Autodesk Inventor part; units mm, degrees
ref_plane "YZ Plane" through (0, 0, 0) normal (1, 0, 0) x (0, 1, 0)
ref_plane "XZ Plane" through (0, 0, 0) normal (0, 1, 0) x (-1, 0, 0)
ref_plane "XY Plane" through (0, 0, 0) normal (0, 0, 1) x (1, 0, 0)
sketch "Sketch1" plane through (0, 0, 0) normal (0, 0, 1) x (1, 0, 0)
  line L0 (-25.4072, 25.3665) -> (76.1928, 25.3665)
  line L1 (76.1928, 25.3665) -> (76.1928, -76.2335)
  line L2 (76.1928, -76.2335) -> (-25.4072, -76.2335)
  line L3 (-25.4072, -76.2335) -> (-25.4072, 25.3665)
  point P0 (0, 0)
  dimension "d0" = 101.6
  dimension "d1" = 101.6
extrude "Extrusion1" add sketch "Sketch1" along normal blind 0.7366
sketch "Sketch2" plane through (0, 0, 0.7366) normal (0, 0, 1) x (1, 0, 0)
  line L0 (-25.4072, 25.3665) -> (76.1928, -76.2335)
  line L1 (76.1928, 25.3665) -> (-25.4072, -76.2335)
  circle A0 centre (25.3928, -25.4335) radius 27.432
  point P0 (0, 0)
  dimension "d4" = 54.864
extrude "Extrusion2" cut sketch "Sketch2" against normal blind 0.7366
sketch "Sketch3" plane through (0, 0, 0.7366) normal (0, 0, 1) x (1, 0, 0)
  line L0 (-25.4072, -76.2335) -> (-25.4072, 25.3665)
  line L1 (-25.4072, 25.3665) -> (-25.4072, -25.4335)
  line L2 (-25.4072, -25.4335) -> (-25.4072, 19.4102)
  line L3 (-25.4072, 25.3665) -> (76.1928, -76.2335)
  line L4 (76.1928, 25.3665) -> (-25.4072, -76.2335)
  circle A0 centre (-19.4509, 19.4102) radius 1.9812
  point P0 (0, 0)
  dimension "d7" = 44.8437
  dimension "d8" = 3.9624
extrude "Extrusion3" cut sketch "Sketch3" against normal blind 0.7366 contours A0 L3 | L3 A0
sketch "Sketch4" plane through (0, 0, 0.7366) normal (0, 0, 1) x (1, 0, 0)
  line L0 (-25.4072, -76.2335) -> (76.1928, 25.3665)
  line L1 (-25.4072, 25.3665) -> (76.1928, -76.2335)
  circle A0 centre (70.2365, 19.4102) radius 1.9819
  circle A1 centre (70.2365, -70.2772) radius 1.983
  circle A2 centre (-19.4509, -70.2772) radius 1.9812
  point P0 (0, 0)
extrude "Extrusion4" cut sketch "Sketch4" against normal blind 0.7366
sketch "Sketch5" plane through (0, 0, 0.7366) normal (0, 0, 1) x (1, 0, 0)
  circle A0 centre (25.3928, -25.4335) radius 27.432
  circle A1 centre (25.3928, -25.4335) radius 29.972
  circle A2 centre (25.3928, -25.4335) radius 32.512
  point P0 (0, 0)
  dimension "d13" = 59.944
  dimension "d14" = 65.024
extrude "Extrusion5" add sketch "Sketch5" along normal blind 6.6548 contours A2
fillet "Fillet1" radius 3.175 4 edges at (-25.4072, 25.3665, 0.3683) (76.1928, 25.3665, 0.3683) (76.1928, -76.2335, 0.3683) (-25.4072, -76.2335, 0.3683)
sketch "Sketch6" plane through (0, 0, 0) normal (0, 0, -1) x (-1, 0, 0)
  circle A0 centre (-70.2365, 19.4102) radius 1.9819
  circle A1 centre (19.4509, -70.2772) radius 1.9812
  circle A2 centre (-70.2365, -70.2772) radius 1.983
  circle A3 centre (19.4509, 19.4102) radius 1.9812
  point P0 (0, 0)
extrude "Extrusion6" add sketch "Sketch6" against normal blind 0.7366
sketch "Sketch7" plane through (0, 0, 0) normal (0, 0, -1) x (-1, 0, 0)
  line L0 (-76.1928, 25.3665) -> (-70.2238, 25.3665)
  line L1 (-70.2238, 25.3665) -> (-70.2238, 19.3975)
  line L2 (-70.2238, 19.3975) -> (-76.1928, 19.3975)
  line L3 (-76.1928, 19.3975) -> (-76.1928, 25.3665)
  line L4 (-76.1928, -76.2335) -> (-70.2238, -76.2335)
  line L5 (-70.2238, -76.2335) -> (-70.2238, -70.2645)
  line L6 (-70.2238, -70.2645) -> (-76.1928, -70.2645)
  line L7 (-76.1928, -70.2645) -> (-76.1928, -76.2335)
  line L8 (25.4072, 25.3665) -> (19.4382, 25.3665)
  line L9 (19.4382, 25.3665) -> (19.4382, 19.3975)
  line L10 (19.4382, 19.3975) -> (25.4072, 19.3975)
  line L11 (25.4072, 19.3975) -> (25.4072, 25.3665)
  line L12 (25.4072, -76.2335) -> (19.4382, -76.2335)
  line L13 (19.4382, -76.2335) -> (19.4382, -70.2645)
  line L14 (19.4382, -70.2645) -> (25.4072, -70.2645)
  line L15 (25.4072, -70.2645) -> (25.4072, -76.2335)
  circle A0 centre (-70.2238, -70.2645) radius 1.9812
  circle A1 centre (-70.2238, 19.3975) radius 1.9812
  circle A2 centre (19.4382, 19.3975) radius 1.9812
  circle A3 centre (19.4382, -70.2645) radius 1.9812
  point P0 (0, 0)
  dimension "d20" = 5.969
  dimension "d21" = 5.969
  dimension "d22" = 5.969
  dimension "d23" = 5.969
  dimension "d24" = 5.969
  dimension "d25" = 3.9624
extrude "Extrusion7" cut sketch "Sketch7" against normal blind 0.7366 contours A1 L2 L1 | L1 L2 A1 | A0 L6 L5 | L5 L6 A0 | A2 L10 L9 | L9 L10 A2 | A3 L14 L13 | L13 L14 A3
properties part number "1"
Verification items for the finished model (mm, model axes). A direction names the side the tool comes from. Give positions to 0.01 mm unless a question says otherwise; leave off trailing zeros. Loops run counter-clockwise (first coordinate to the right, second up) from the corner with the lowest first, then second, coordinate; pieces in that order, holes last.
1) Thickness scan on line 1 along Y through (x, z) = (25.5, 4.75); line 2 along Z through (x, y) = (45.5, -63.5); line 3 along Y through (x, z) = (-1.5, 3). Record the ranges inside material, lowest first.
2) Draft check along Y on faces 3 (the cylindrical face through (75.238, -75.328, 0.373)), 4 (the flat face through (-4, -18, 7.391)), 5 (the cylindrical face through (75.3, 24.4, 0.4)), 6 (the cylindrical face through (69.31, -72.022, 0.363)). Enter one of: pulls with the +Y half, pulls with the -Y half, needs draft (parallel to the pull), parting line crosses it, or undercut.
3) Depth check by flat-ended pin: pin 1 Ø3 at (x, z) = (7.5, 3.5) entering from +Y; pin 2 Ø2 at (y, z) = (-49, 5.5) entering from -X; pin 3 Ø6.5 at (x, y) = (-19.44, 19.4) entering from +Z; pin 4 Ø5 at (x, y) = (-9.5, -33.5) entering from -Z. Enter the tip coordinate at first touch or a pass-through.
4) Sectioned sample at B-B, the plane x = 48.5. Enter the section's corners in (y, z).
5) Sectioned sample at C-C, the plane z = 5. Enter the section's corners in (x, y), then the cut area to 3 significant figures.
6) Sectioned sample at D-D, the plane y = 16. Enter the section's corners in (x, z).
7) Set-up check for faces 1 (the cylindrical face through (-24.452, 24.461, 0.373)), 2 (the cylindrical face through (18.895, 3.826, 4.017)): record each of +Z, -Z, +X, -X, +Y, -Y from which the full face is reachable in a straight line by a thin tool's end or side.
8) Sectioned sample at A-A, the plane y = -34. Enter the section's corners in (x, z), then the cut area to 3 significant figures.
Answers:
1. line 1: y = -57.95 to -55.41, 4.54 to 7.08
1. line 2: z = 0 to 0.74
1. line 3: y = -43.7 to -38.67, -12.2 to -7.16
2. face 3: pulls with the -Y half
2. face 4: needs draft
2. face 5: pulls with the +Y half
2. face 6: undercut
3. pin 1: stops at y = 2.64
3. pin 2: stops at x = 1.99
3. pin 3: stops at z = 0.74
3. pin 4: stops at z = 0
4. outline: (-76.23, 0) - (-40.22, 0) - (-40.22, 0.74) - (-44.52, 0.74) - (-44.52, 7.39) - (-48.3, 7.39) - (-48.3, 0.74) - (-76.23, 0.74) - close; (-10.65, 0) - (25.37, 0) - (25.37, 0.74) - (-2.56, 0.74) - (-2.56, 7.39) - (-6.34, 7.39) - (-6.34, 0.74) - (-10.65, 0.74) - close
5. outline: circle Ø65.02 at (25.39, -25.43); hole circle Ø59.94 at (25.39, -25.43)
5. area: 499 mm2
6. outline: (-25.41, 0) - (76.19, 0) - (76.19, 0.74) - (-25.41, 0.74) - close
7. face 1: +Z, -Z, -X, +Y
7. face 2: +Z
8. outline: (-25.41, 0) - (-0.67, 0) - (-0.67, 0.74) - (-3.33, 0.74) - (-3.33, 7.39) - (-5.97, 7.39) - (-5.97, 0.74) - (-25.41, 0.74) - close; (51.45, 0) - (76.19, 0) - (76.19, 0.74) - (56.76, 0.74) - (56.76, 7.39) - (54.11, 7.39) - (54.11, 0.74) - (51.45, 0.74) - close
8. area: 71.6 mm2
